from build123d import *

# Parameters (mm, degrees)
SKETCH_1_W          = 44.92820323
SKETCH_1_H          = 44.928203231
EXTRUDE_1_DEPTH     = 9
SKETCH_2_W          = 126.5
SKETCH_2_H          = 82.5
SKETCH_2_W_2        = 44.92820323
SKETCH_2_H_2        = 44.928203231
EXTRUDE_2_DEPTH     = 5
CHAMFER_1_SIZE      = 2
CHAMFER_1_SIZE2     = 11.342563639
EXTRUDE_3_DEPTH     = 10
SKETCH_4_W          = 20
SKETCH_4_H          = 16
SKETCH_4_R          = 2.2
EXTRUDE_4_DEPTH     = 4
EXTRUDE_5_DEPTH     = 20
EXTRUDE_6_DEPTH     = 20
SKETCH_7_W          = 14
SKETCH_7_H          = 13
CUT_EXTRUDE_1_DEPTH = 20
EXTRUDE_7_DEPTH     = 3
EXTRUDE_8_DEPTH     = 3
CHAMFER_2_SIZE      = 3
SKETCH_10_W         = 1
SKETCH_10_H         = 16
SKETCH_10_H_2       = 15.995398116
CUT_EXTRUDE_2_DEPTH = 9


with BuildPart() as part:
    # Эскиз1 → Бобышка-Вытянуть1 (new body)
    with BuildSketch(Plane(origin=(0, 122.195974268, 0), x_dir=(1, 0, 0), z_dir=(0, 1, 0))):
        Polygon((16.558980694, -48.273129836), (16.558980694, -54.273129836), (7.558980694, -63.273129836), (1.558980694, -63.273129836), (1.558980694, -115.773129836), (7.558980694, -115.773129836), (16.558980694, -124.773129836), (16.558980694, -130.773129836), (113.058980694, -130.773129836), (113.058980694, -124.773129836), (122.058980694, -115.773129836), (128.058980694, -115.773129836), (128.058980694, -63.273129836), (122.058980694, -63.273129836), (113.058980694, -54.273129836), (113.058980694, -48.273129836), align=None)
        with Locations((64.808980694, -89.523129837)):
            Rectangle(SKETCH_1_W, SKETCH_1_H, mode=Mode.SUBTRACT)
    extrude(amount=EXTRUDE_1_DEPTH)

    # Эскиз2 → Бобышка-Вытянуть2 (add)
    with BuildSketch(Plane(origin=(0, 131.195974268, 0), x_dir=(1, 0, 0), z_dir=(0, 1, 0))):
        with Locations((64.808980694, -89.523129836)):
            Rectangle(SKETCH_2_W, SKETCH_2_H)
        with Locations((64.808980694, -89.523129837)):
            Rectangle(SKETCH_2_W_2, SKETCH_2_H_2, mode=Mode.SUBTRACT)
    extrude(amount=EXTRUDE_2_DEPTH)

    # Фаска1
    chamfer_1_edges = [part.edges().sort_by_distance(p)[0] for p in [
        (64.808980694, 136.195974268, 67.059028221),
        (42.344879079, 136.195974268, 89.523129836),
        (64.808980694, 136.195974268, 111.987231452),
        (87.273082309, 136.195974268, 89.523129836),
    ]]
    chamfer_1_side = [part.faces().sort_by_distance(p)[0] for p in [
        (64.808980694, 136.195974268, 49.78337816),
    ]]
    chamfer(chamfer_1_edges, length=CHAMFER_1_SIZE, length2=CHAMFER_1_SIZE2, reference=chamfer_1_side[0])

    # Эскиз3 → Бобышка-Вытянуть3 (add)
    with BuildSketch(Plane(origin=(0, 136.195974268, 0), x_dir=(1, 0, 0), z_dir=(0, 1, 0))):
        Polygon((128.058980694, -68.073129836), (128.058980694, -48.273129836), (108.258980694, -48.273129836), (108.258980694, -56.073129836), (123.258980694, -56.073129836), (123.258980694, -68.073129836), align=None)
        Polygon((21.358980694, -48.273129836), (1.558980694, -48.273129836), (1.558980694, -68.073129836), (6.358980694, -68.073129836), (6.358980694, -56.073129836), (21.358980694, -56.073129836), align=None)
        Polygon((128.058980694, -110.973129836), (128.058980694, -130.773129836), (108.258980694, -130.773129836), (108.258980694, -122.973129836), (123.258980694, -122.973129836), (123.258980694, -110.973129836), align=None)
    extrude(amount=EXTRUDE_3_DEPTH)

    # Эскиз4 → Бобышка-Вытянуть4 (add)
    # profile 1 of 3: a face of its own
    with BuildSketch(Plane(origin=(0, 146.195974268, 0), x_dir=(1, 0, 0), z_dir=(0, 1, 0))):
        with Locations((118.058980694, -138.773129836)):
            Rectangle(SKETCH_4_W, SKETCH_4_H)
        with Locations(Location((120.058980694, -138.773129836, 0), (0, 0, 180))):
            Circle(SKETCH_4_R, mode=Mode.SUBTRACT)
    # profile 2 of 3: a face of its own
    with BuildSketch(Plane(origin=(0, 146.195974268, 0), x_dir=(1, 0, 0), z_dir=(0, 1, 0))):
        Polygon((128.058980694, -48.273129836), (128.058980694, -32.273129836), (108.058980694, -32.273129836), (108.258980694, -48.273129836), align=None)
        with Locations(Location((120.058980694, -40.273129836, 0), (0, 0, 180))):
            Circle(SKETCH_4_R, mode=Mode.SUBTRACT)
    # profile 3 of 3: a face of its own
    with BuildSketch(Plane(origin=(0, 146.195974268, 0), x_dir=(1, 0, 0), z_dir=(0, 1, 0))):
        Polygon((1.558980694, -48.273129836), (1.558980694, -32.273129836), (21.558980694, -32.273129836), (21.358980694, -48.273129836), align=None)
        with Locations(Location((11.558980694, -40.273129836, 0), (0, 0, 180))):
            Circle(SKETCH_4_R, mode=Mode.SUBTRACT)
    extrude(amount=-EXTRUDE_4_DEPTH)

    # Эскиз5 → Бобышка-Вытянуть5 (add)
    with BuildSketch(Plane(origin=(128.058980694, 0, 0), x_dir=(0, 0, -1), z_dir=(1, 0, 0))):
        Polygon((-146.773129836, 142.195974268), (-130.773129836, 142.195974268), (-130.773129836, 131.195974268), (-131.773129836, 131.195974268), (-131.773129836, 122.195974268), align=None)
        Polygon((-32.273129836, 142.195974268), (-48.273129836, 142.195974268), (-48.273129836, 131.195974268), (-47.273129836, 131.195974268), (-47.273129836, 122.195974268), align=None)
    extrude(amount=-EXTRUDE_5_DEPTH)

    # Эскиз6 → Бобышка-Вытянуть6 (add)
    with BuildSketch(Plane.ZY.offset(-1.558980694)):
        Polygon((32.273129836, 142.195974268), (48.273129836, 142.195974268), (48.273129836, 131.195974268), (47.273129836, 131.195974268), (47.273129836, 122.195974268), align=None)
    extrude(amount=-EXTRUDE_6_DEPTH)

    # Эскиз7 → Вырез-Вытянуть1 (cut)
    with BuildSketch(Plane(origin=(0, 122.195974268, 0), x_dir=(-1, 0, 0), z_dir=(0, -1, 0))):
        with Locations((-11.558980694, -38.773129836)):
            Rectangle(SKETCH_7_W, SKETCH_7_H)
        with Locations((-118.058980694, -38.773129836)):
            Rectangle(SKETCH_7_W, SKETCH_7_H)
        with Locations((-118.058980694, -140.273129836)):
            Rectangle(SKETCH_7_W, SKETCH_7_H)
    extrude(amount=-CUT_EXTRUDE_1_DEPTH, mode=Mode.SUBTRACT)

    # Эскиз8 → Бобышка-Вытянуть7 (add)
    with BuildSketch(Plane(origin=(128.058980694, 0, 0), x_dir=(0, 0, -1), z_dir=(1, 0, 0))):
        Polygon((-142.273129836, 136.195974268), (-36.773129836, 136.195974268), (-47.273129836, 122.195974268), (-131.768527952, 122.195974268), align=None)
    extrude(amount=EXTRUDE_7_DEPTH)

    # Эскиз9 → Бобышка-Вытянуть8 (add)
    with BuildSketch(Plane.ZY.offset(-1.558980694)):
        Polygon((47.296106509, 122.195974268), (36.773129836, 136.195974268), (130.773129836, 136.195974268), (130.773129836, 122.195974268), align=None)
    extrude(amount=EXTRUDE_8_DEPTH)

    # Фаска2
    chamfer_2_edges = [part.edges().sort_by_distance(p)[0] for p in [
        (131.058980694, 136.195974268, 89.523129836),
        (-1.441019306, 136.195974268, 83.773129836),
    ]]
    chamfer(chamfer_2_edges, length=CHAMFER_2_SIZE - 0.0001)  # a hair under: the kernel refuses the full size

    # Эскиз10 → Вырез-Вытянуть2 (cut)
    with BuildSketch(Plane(origin=(0, 122.195974268, 0), x_dir=(-1, 0, 0), z_dir=(0, -1, 0))):
        with Locations((-128.558980694, -55.273129836)):
            Rectangle(SKETCH_10_W, SKETCH_10_H)
        with Locations((-128.558980694, -123.770828894)):
            Rectangle(SKETCH_10_W, SKETCH_10_H_2)
        Polygon((-1.558980694, -47.273129836), (-1.558980694, -63.273129836), (-0.558980694, -63.273129836), (-0.558980694, -47.296106509), align=None)
    extrude(amount=-CUT_EXTRUDE_2_DEPTH, mode=Mode.SUBTRACT)


solid = part.part
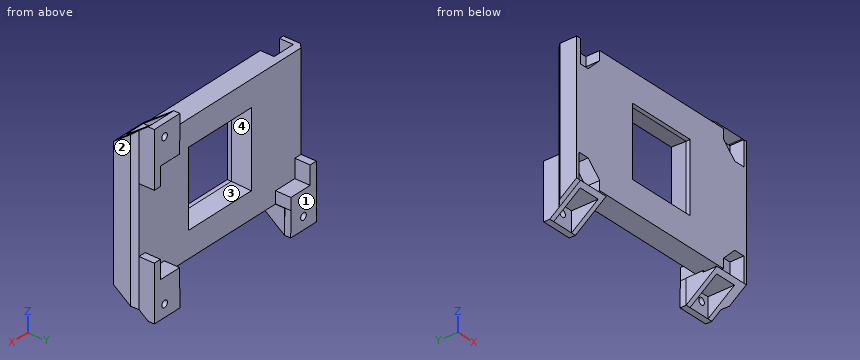
For this review, take the finished solid that the model builds, in its own axes (mm). Face numbers are marked on the shaded views. Give positions to 0.01 mm unless a question says otherwise; leave off trailing zeros. Order: outer loops, then holes, each group sorted by start corner. A loop starts at its lowest first (then second) coordinate and runs counter-clockwise, first axis right, second up. Notation, with made-up numbers: (41, 56.25) - (100, 56.25) arc R27 ccw to (100, 92.25) - close; hole circle Ø8 at (73.25, -16). An arc over 180 degrees is marked (long way). Answer as a JSON object with one key per item and string values. Group by question number.
Item 1: Take a section at C-C on y = 144.5. Give the boundary of the cut face in (x, z), and give its area (3 significant figures).
Item 2: Clearance check with flat-ended pins moving along their axes: pin 1 Ø10 at (x, y) = (85.5, 129) entering from +Z; pin 2 Ø4.5 at (x, y) = (120.5, 126.5) entering from -Z; pin 3 Ø10 at (x, y) = (85, 132) entering from -Z; pin 4 Ø10.5 at (y, z) = (132.5, 39.5) entering from -X. State where each tip first meets the part, or that it passes through.
Item 3: Take a section at B-B on x = 46. Give the boundary of the cut face in (y, z).
Item 4: Take a section at A-A on z = 82. Give the boundary of the cut face in (x, y), and give its area (3 significant figures).
Item 5: Draft analysis for pull direction X (two halves, no side actions). For the marked faces 1, 2, 3 and 4, state which applies: pulls with the +X half, pulls with the -X half, needs draft (parallel to the pull), parting line crosses it, or undercut.
Item 6: Wall thickness on line 1 along X through (y, z) = (132.25, 42.5); line 2 along X through (y, z) = (126.5, 128); line 3 along X through (y, z) = (143.75, 51): over which ranges is each line inside the solid? List them lowest first.
Reported:
{
 "1": {"outline": "(1.56, 32.27) - (21.56, 32.27) - (21.36, 48.27) - (21.36, 56.07) - (6.36, 56.07) - (6.36, 68.07) - (1.56, 68.07) - close; (108.06, 32.27) - (128.06, 32.27) - (128.06, 68.07) - (123.26, 68.07) - (123.26, 56.07) - (108.26, 56.07) - (108.26, 48.27) - close; (108.06, 130.77) - (108.26, 130.77) - (108.26, 122.97) - (123.26, 122.97) - (123.26, 110.97) - (128.06, 110.97) - (128.06, 146.77) - (108.06, 146.77) - close; hole circle Ø4.4 at (11.56, 40.27); hole circle Ø4.4 at (120.06, 40.27); hole circle Ø4.4 at (120.06, 138.77)", "area": "1,550 mm^2"},
 "2": {"pin 1": "z = 130.77", "pin 2": "z = 45.27", "pin 3": "z = 48.27", "pin 4": "x = -1.44"},
 "3": {"outline": "(122.2, 48.27) - (136.2, 48.27) - (136.2, 65.06) - (124.85, 67.06) - (122.2, 67.06) - close; (122.2, 111.99) - (124.85, 111.99) - (136.2, 113.99) - (136.2, 130.77) - (122.2, 130.77) - close"},
 "4": {"outline": "(-1.44, 122.2) - (42.34, 122.2) - (42.34, 124.85) - (40.34, 136.2) - (1.56, 136.2) - (-1.44, 133.2) - close; (87.27, 122.2) - (131.06, 122.2) - (131.06, 133.2) - (128.06, 136.2) - (89.27, 136.2) - (87.27, 124.85) - close", "area": "1,190 mm^2"},
 "5": {"face 1": "needs draft", "face 2": "pulls with the +X half", "face 3": "undercut", "face 4": "undercut"},
 "6": {"line 1": "-1.44 to 4.56, 18.56 to 21.56, 108.06 to 111.06, 125.06 to 131.06", "line 2": "-1.44 to 1.56, 16.56 to 113.06, 129.06 to 131.06", "line 3": "1.56 to 21.36, 108.26 to 128.06"}
}
